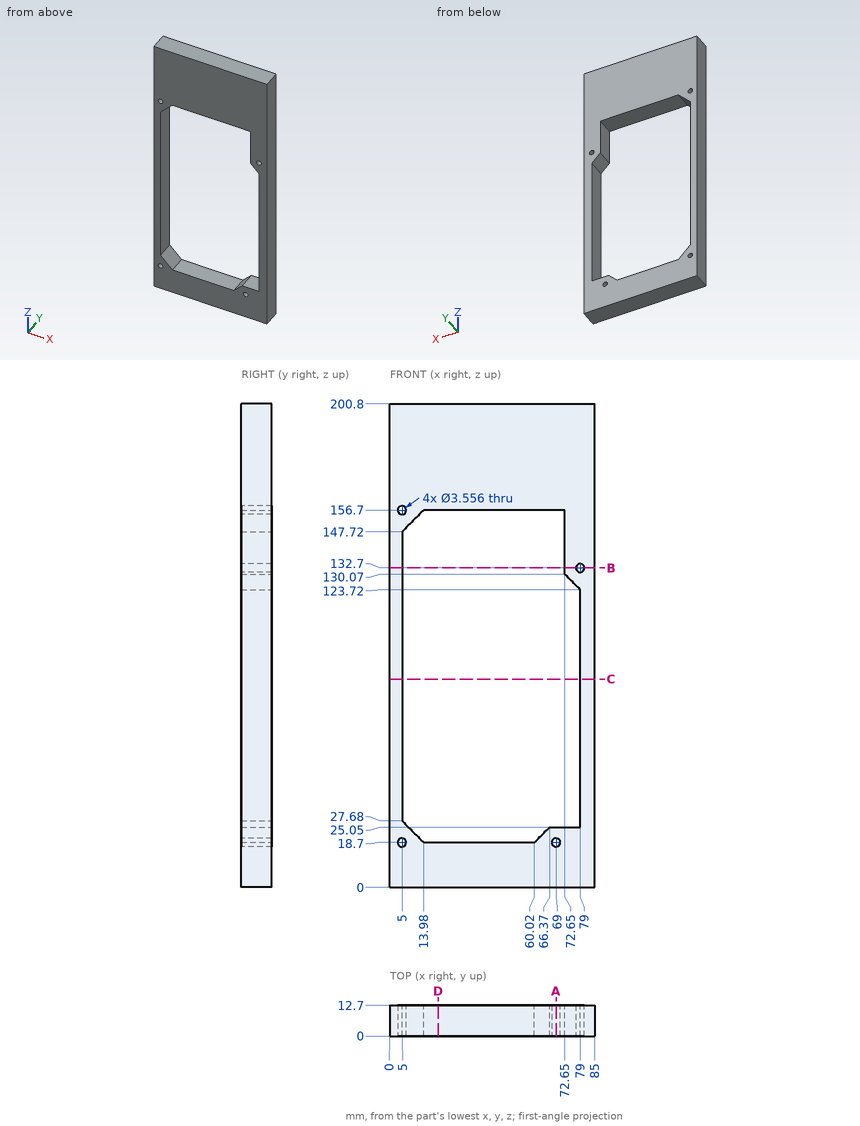
Drawing for the job (mm, zero at the part's lowest x, y, z). Round coordinates to 2 decimals unless told otherwise and drop trailing zeros. Loops run counter-clockwise (first coordinate to the right, second up) from the corner with the lowest first, then second, coordinate; pieces in that order, holes last.
1. Wall check: probe 1 along X at (y, z) = (2.5, 132.7); probe 2 along X at (y, z) = (10.75, 68.5); probe 3 along Z at (x, y) = (41, 4.5). Give the ranges that are in metal, low to high.
Check values:
probe 1: x = 0 to 5, 72.65 to 77.22, 80.78 to 85
probe 2: x = 0 to 5, 79 to 85
probe 3: z = 0 to 18.7, 156.7 to 200.8
2. Band-saw the part on D-D, the plane x = 20. List the corners of the cut face in (y, z).
Check values:
outline: (0, 0) - (12.7, 0) - (12.7, 18.7) - (0, 18.7) - close; (0, 156.7) - (12.7, 156.7) - (12.7, 200.8) - (0, 200.8) - close
3. Band-saw the part on C-C, the plane z = 86.5. List the corners of the cut face in (x, y), and give its area (3 significant figures).
Check values:
outline: (0, 0) - (5, 0) - (5, 12.7) - (0, 12.7) - close; (79, 0) - (85, 0) - (85, 12.7) - (79, 12.7) - close
area: 140 mm2
4. Band-saw the part on B-B, the plane z = 132.7. List the corners of the cut face in (x, y).
Check values:
outline: (0, 0) - (5, 0) - (5, 12.7) - (0, 12.7) - close; (72.65, 0) - (77.22, 0) - (77.22, 12.7) - (72.65, 12.7) - close; (80.78, 0) - (85, 0) - (85, 12.7) - (80.78, 12.7) - close
5. Drop a flat-ended pin along its axis: P1, Ø2, axis at x = 5, z = 18.7, coming from the +Y side. Give the stop position or say it passes through.
Check values:
P1: passes through
6. Band-saw the part on A-A, the plane x = 69. List the corners of the cut face in (y, z), and give its area (3 significant figures).
Check values:
outline: (0, 0) - (12.7, 0) - (12.7, 16.92) - (0, 16.92) - close; (0, 20.48) - (12.7, 20.48) - (12.7, 25.05) - (0, 25.05) - close; (0, 156.7) - (12.7, 156.7) - (12.7, 200.8) - (0, 200.8) - close
area: 833 mm2
